```python
from build123d import *


with BuildPart() as f2:
    # F2: sweep along a path in F1
    with BuildLine(Plane.XZ) as f2_path:
        Line((0, 0), (0, 95.25))
        ThreePointArc((0, 95.25), (1.859872, 99.740128), (6.35, 101.6))
        Line((6.35, 101.6), (25.4, 101.6))
    # F0 (on Top) → F2 (sweep)
    with BuildSketch(Plane.XY):
        Polygon((0.916544, 1.5875), (-0.916544, 1.5875), (-1.833087, 0), (-0.916544, -1.5875), (0.916544, -1.5875), (1.833087, 0), align=None)
    sweep(path=f2_path.line)


solid = f2.part
```
Could you check a few things on this model? Use its own coordinates, in mm. Give positions to 0.01 mm unless a question says otherwise; leave off trailing zeros. Loops run counter-clockwise (first coordinate to the right, second up) from the corner with the lowest first, then second, coordinate; pieces in that order, holes last. Notation, with made-up numbers: (-8, 77.25) -> (50, 77.25) arc R8 ccw to (50, 88.25) -> close; hole circle Ø5 at (-39.75, 81.5). An arc over 180 degrees is marked (long way). Put each result on its own line as item: value.
(1) Imagine slicing it at A-A on y = -0.5. Write out the boundary of the cut face in (x, z).
Computed:
outline: (-1.54, 0) -> (1.54, 0) -> (1.54, 95.25) arc R4.81 cw to (6.35, 100.06) -> (25.4, 100.06) -> (25.4, 103.14) -> (6.35, 103.14) arc R7.89 ccw to (-1.54, 95.25) -> close
(2) Imagine slicing it at C-C on x = 15. Write out the boundary of the cut face in (y, z).
Computed:
outline: (-1.59, 100.68) -> (0, 99.77) -> (1.59, 100.68) -> (1.59, 102.52) -> (0, 103.43) -> (-1.59, 102.52) -> close
(3) Please list where these lines run through material, in increasing order: probe 1 along X at (y, z) = (0, 43.5); probe 2 along X at (y, z) = (-0.45, 5); probe 3 along Z at (x, y) = (22.5, 0.25). Write a range as [from, to].
Computed:
probe 1: [-1.83, 1.83]
probe 2: [-1.57, 1.57]
probe 3: [99.91, 103.29]
(4) I'm going to push a flat-ended pin straight in: pin 1 Ø1.5 at (y, z) = (1, 33) entering from +X. Where does the tip first touch, or does it pass through?
Computed:
pin 1: x = 1.69
(5) Imagine slicing it at B-B on z = 64. Write out the boundary of the cut face in (x, y), plus the area to 3 significant figures.
Computed:
outline: (-1.83, 0) -> (-0.92, -1.59) -> (0.92, -1.59) -> (1.83, 0) -> (0.92, 1.59) -> (-0.92, 1.59) -> close
area: 8.73 mm^2
